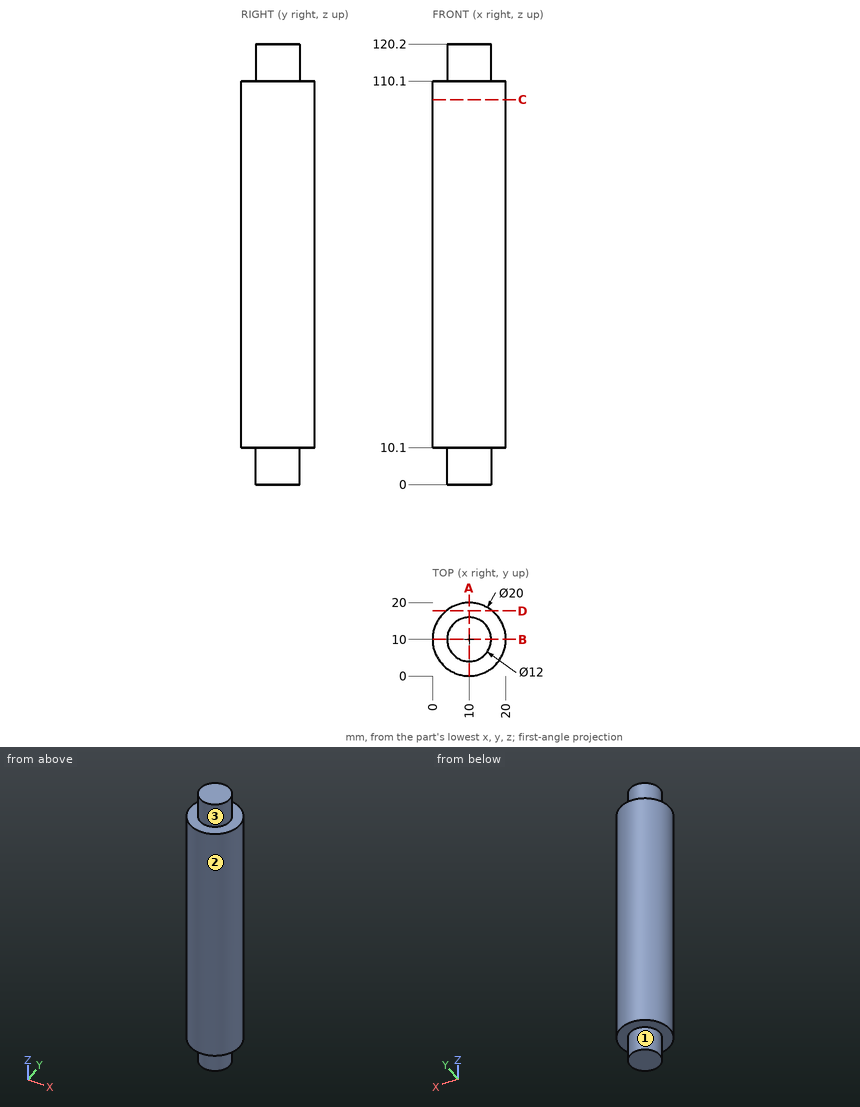
Can you work these out from the drawing? Everything is in mm from the part's minimum corner. A direction names the side the tool comes from. Give positions to 0.01 mm unless a question says otherwise; leave off trailing zeros. Order: outer loops, then holes, each group sorted by start corner. A loop starts at its lowest first (then second) coordinate and runs counter-clockwise, first axis right, second up. Notation, with made-up numbers: M -10.5,78 L 4.5,78 A11 ccw 4.5,90 Z; hole C 80,49.5 d5. An arc over 180 degrees is marked long. Use a Markdown table: item, result. Add a question column.
Item 1: For the marked faces 1, 2 and 3, which set-ups out of +Z, -Z, +X, -X, +Y, -Y let a thin tool reach every point of the face, with its end or its side?
Item 2: If I drill on L1, parallel to X at y = 9.5, z = 14; L2, parallel to Z at x = 16.5, y = 11.5; L3, parallel to X at y = 18, z = 87, over which ranges is the centre line in solid material (lowest first)? Write a range as [from, to].
Item 3: Suppose I cut it at D-D (y = 17.75). List the corners of the cut face in (x, z) for me, then the cut area to 3 significant figures.
Item 4: Will these pins go through, and if not, where does the flat tip stop? pin 1 (1 mm diameter, centred on x = 6, y = 4.5, fed in from -Z); pin 2 (4 mm diameter, centred on y = 6, z = 83.5, fed in from -X); pin 3 (1.5 mm diameter, centred on y = 6, z = 40.5, fed in from +X).
Item 5: Suppose I cut it at C-C (z = 105). List the corners of the cut face in (x, y) for me, then the cut area to 3 significant figures.
Item 6: Suppose I cut it at A-A (x = 10). List the corners of the cut face in (y, z) for me, then the cut area to 3 significant figures.
Answer sheet:
| question | item | result |
|---|---|---|
| 1 | face 1 | -Z |
| 1 | face 2 | +Z, -Z |
| 1 | face 3 | +Z |
| 2 | L1 | x = [0.01, 19.99] |
| 2 | L2 | z = [10.1, 110.1] |
| 2 | L3 | x = [4, 16] |
| 3 | outline | M 3.68,10.1 L 16.32,10.1 L 16.32,110.1 L 3.68,110.1 Z |
| 3 | area | 1,260 mm² |
| 4 | pin 1 | stops at z = 10.1 |
| 4 | pin 2 | stops at x = 0.2 |
| 4 | pin 3 | stops at x = 19.46 |
| 5 | outline | C 10,10 d20 |
| 5 | area | 314 mm² |
| 6 | outline | M 0,10.1 L 4,10.1 L 4,0 L 16,0 L 16,10.1 L 20,10.1 L 20,110.1 L 16,110.1 L 16,120.2 L 4,120.2 L 4,110.1 L 0,110.1 Z |
| 6 | area | 2,240 mm² |
